from build123d import *

# Parameters (mm, degrees)
SKETCH2_R                      = 250
BOSS_EXTRUDE1_DEPTH            = 300
CUT_EXTRUDE1_DEPTH             = 464.680924775
CUT_EXTRUDE1_DEPTH_BACK        = 464.680924775
SKETCH3_W                      = 380
SKETCH3_H                      = 55
SHELL1_START                   = 140
SHELL1_OUTLINE_R               = 240
SHELL1_DEPTH                   = 150
SHELL1_START_2                 = 10
SHELL1_2_OUTLINE_R             = 240
SHELL1_2_DEPTH                 = 55
SHELL1_START_3                 = 65
SHELL1_3_DEPTH                 = 75
CUT_EXTRUDE2_REACH             = 546.885
SKETCH4_W                      = 120
SKETCH4_H                      = 20
CUT_EXTRUDE5_START             = -20
SKETCH6_R                      = 240
CUT_EXTRUDE5_DEPTH             = 20
CUT_EXTRUDE6_REACH             = 465.681
SKETCH8_3_W                    = 50
SKETCH8_3_H                    = 20
CUT_EXTRUDE6_DIRECTION_2_DEPTH = 464.680924775
CIRPATTERN1_COUNT              = 2
CIRPATTERN1_ANGLE              = 90
FILLET2_R                      = 30


# Read off the part's stored shape, not the designer's step: Shell1
with BuildPart() as part:
    # Sketch2 → Boss-Extrude1 (new body)
    with BuildSketch(Plane(origin=(0, 0, 0), x_dir=(1, 0, 0), z_dir=(0, 1, 0))):
        with Locations(Location((0, 0, 0), (0, 0, 270))):
            Circle(SKETCH2_R)
    extrude(amount=BOSS_EXTRUDE1_DEPTH)

    # Sketch3 → Cut-Extrude1 (cut, two sides: drawn at the far end of the back side and taken through both)
    with BuildSketch(Plane.XY.offset(-CUT_EXTRUDE1_DEPTH_BACK)):
        with Locations((-60, 102.5)):
            Rectangle(SKETCH3_W, SKETCH3_H)
    extrude(amount=CUT_EXTRUDE1_DEPTH + CUT_EXTRUDE1_DEPTH_BACK, mode=Mode.SUBTRACT)

    # Shell1 outline → Shell1 (cut)
    with BuildSketch(Plane(origin=(0, 0, 0), x_dir=(1, 0, 0), z_dir=(0, 1, 0)).offset(SHELL1_START)):
        Circle(SHELL1_OUTLINE_R)
    extrude(amount=SHELL1_DEPTH, mode=Mode.SUBTRACT)

    # Shell1 2 outline → Shell1 2 (cut)
    with BuildSketch(Plane(origin=(0, 0, 0), x_dir=(1, 0, 0), z_dir=(0, 1, 0)).offset(SHELL1_START_2)):
        Circle(SHELL1_2_OUTLINE_R)
    extrude(amount=SHELL1_2_DEPTH, mode=Mode.SUBTRACT)

    # Shell1 3 outline → Shell1 3 (cut)
    with BuildSketch(Plane(origin=(0, 0, 0), x_dir=(1, 0, 0), z_dir=(0, 1, 0)).offset(SHELL1_START_3)):
        with BuildLine():
            ThreePointArc((140, -194.935886896), (240, 0), (140, 194.935886896))
            Line((140, 194.935886896), (140, -194.935886896))
        make_face()
    extrude(amount=SHELL1_3_DEPTH, mode=Mode.SUBTRACT)

    # Sketch4 → Cut-Extrude2 (cut, up to next)
    with BuildSketch(Plane.ZY.offset(-130), mode=Mode.PRIVATE) as cut_extrude2_sk1:
        with Locations((0, 102.5)):
            Rectangle(SKETCH4_W, SKETCH4_H)
    cut_extrude2_tool1 = extrude(cut_extrude2_sk1.sketch, amount=-CUT_EXTRUDE2_REACH, mode=Mode.PRIVATE) & part.part
    add(cut_extrude2_tool1.solids().sort_by_distance((130, 102.5, 0))[0], mode=Mode.SUBTRACT)

    # Sketch6 → Cut-Extrude5 (cut)
    with BuildSketch(Plane(origin=(0, 300, 0), x_dir=(1, 0, 0), z_dir=(0, 1, 0)).offset(CUT_EXTRUDE5_START)):
        with Locations(Location((0, 0, 0), (0, 0, 270))):
            Circle(SKETCH6_R)
    extrude(amount=CUT_EXTRUDE5_DEPTH, mode=Mode.SUBTRACT)

    # Sketch8<3> → Cut-Extrude6 (cut, up to next)
    with BuildSketch(Plane(origin=(0, 0, 0), x_dir=(0, 0, -1), z_dir=(1, 0, 0)), mode=Mode.PRIVATE) as cut_extrude6_sk1:
        with Locations((0, 250)):
            Rectangle(SKETCH8_3_W, SKETCH8_3_H)
    cut_extrude6_tool1 = extrude(cut_extrude6_sk1.sketch, amount=-CUT_EXTRUDE6_REACH, mode=Mode.PRIVATE) & part.part
    cut_extrude6 = cut_extrude6_tool1.solids().sort_by_distance((0, 250, 0))[0]
    add(cut_extrude6, mode=Mode.SUBTRACT)

    # Sketch8<3> → Cut-Extrude6 direction 2 (cut)
    with BuildSketch(Plane(origin=(0, 0, 0), x_dir=(0, 0, -1), z_dir=(1, 0, 0))):
        with Locations((0, 250)):
            Rectangle(SKETCH8_3_W, SKETCH8_3_H)
    cut_extrude6_direction_2 = extrude(amount=CUT_EXTRUDE6_DIRECTION_2_DEPTH, mode=Mode.SUBTRACT)

    # CirPattern1: Cut-Extrude6, Cut-Extrude6 direction 2 ×2 about axis
    cirpattern1_axis = Axis((0, 300, 0), (0, 1, 0))
    add([cut_extrude6.rotate(cirpattern1_axis, i * CIRPATTERN1_ANGLE / (CIRPATTERN1_COUNT - 1)) for i in range(1, CIRPATTERN1_COUNT)], mode=Mode.SUBTRACT)
    add([cut_extrude6_direction_2.rotate(cirpattern1_axis, i * CIRPATTERN1_ANGLE / (CIRPATTERN1_COUNT - 1)) for i in range(1, CIRPATTERN1_COUNT)], mode=Mode.SUBTRACT)

    # Fillet2
    # the kernel refuses this fillet: 30 mm, written as the material it adds along each edge
    with BuildSketch(Plane(origin=(130, 130, -288.541565041), x_dir=(0, -1, 0), z_dir=(0, 0, 1))) as fillet2_piece_1_section:
        with BuildLine():
            CenterArc((FILLET2_R, -FILLET2_R), FILLET2_R, 90, 90)
            Line((0, -FILLET2_R), (0, 0))
            Line((0, 0), (FILLET2_R, 0))
        make_face()
    fillet2_piece_1 = extrude(amount=577.083130081, mode=Mode.PRIVATE)
    fillet2_piece_1 = fillet2_piece_1 & Plane(origin=(0, 108.141191738, 0), x_dir=(0, 0, 1), z_dir=(0, -1, 0)) * Cylinder(250, 1275, mode=Mode.PRIVATE)
    fillet2_piece_1 = split(fillet2_piece_1, bisect_by=Plane(origin=(129.633192853, 108.141191738, -60), z_dir=(0, 0, -1)), keep=Keep.TOP, mode=Mode.PRIVATE)
    fillet2_piece_1 = split(fillet2_piece_1, bisect_by=Plane(origin=(129.633192853, 112.5, -136.881350588), z_dir=(0, -1, 0)), keep=Keep.TOP, mode=Mode.PRIVATE)
    add(fillet2_piece_1)
    with BuildSketch(Plane(origin=(130, 130, -288.541565041), x_dir=(0, -1, 0), z_dir=(0, 0, 1))) as fillet2_piece_2_section:
        with BuildLine():
            CenterArc((FILLET2_R, -FILLET2_R), FILLET2_R, 90, 90)
            Line((0, -FILLET2_R), (0, 0))
            Line((0, 0), (FILLET2_R, 0))
        make_face()
    fillet2_piece_2 = extrude(amount=577.083130081, mode=Mode.PRIVATE)
    fillet2_piece_2 = fillet2_piece_2 & Plane(origin=(0, 124.602125162, 0), x_dir=(0, 0, 1), z_dir=(0, -1, 0)) * Cylinder(250, 1275, mode=Mode.PRIVATE)
    fillet2_piece_2 = split(fillet2_piece_2, bisect_by=Plane(origin=(122.496617269, 124.602125162, -60), z_dir=(0, 0, -1)), keep=Keep.TOP, mode=Mode.PRIVATE)
    fillet2_piece_2 = split(fillet2_piece_2, bisect_by=Plane(origin=(122.496617269, 112.5, -138.903095836), z_dir=(0, 1, 0)), keep=Keep.TOP, mode=Mode.PRIVATE)
    add(fillet2_piece_2)
    with BuildSketch(Plane(origin=(130, 130, -288.541565041), x_dir=(0, -1, 0), z_dir=(0, 0, 1))) as fillet2_piece_3_section:
        with BuildLine():
            CenterArc((FILLET2_R, -FILLET2_R), FILLET2_R, 90, 90)
            Line((0, -FILLET2_R), (0, 0))
            Line((0, 0), (FILLET2_R, 0))
        make_face()
    fillet2_piece_3 = extrude(amount=577.083130081, mode=Mode.PRIVATE)
    fillet2_piece_3 = split(fillet2_piece_3, bisect_by=Plane(origin=(122.639576661, 124.541490092, -60), z_dir=(0, 0, 1)), keep=Keep.TOP, mode=Mode.PRIVATE)
    fillet2_piece_3 = split(fillet2_piece_3, bisect_by=Plane(origin=(122.639576661, 124.541490092, 60), z_dir=(0, 0, -1)), keep=Keep.TOP, mode=Mode.PRIVATE)
    fillet2_piece_3 = split(fillet2_piece_3, bisect_by=Plane(origin=(122.639576661, 112.5, 0), z_dir=(0, 1, 0)), keep=Keep.TOP, mode=Mode.PRIVATE)
    add(fillet2_piece_3)
    with BuildSketch(Plane(origin=(130, 130, -288.541565041), x_dir=(0, -1, 0), z_dir=(0, 0, 1))) as fillet2_piece_4_section:
        with BuildLine():
            CenterArc((FILLET2_R, -FILLET2_R), FILLET2_R, 90, 90)
            Line((0, -FILLET2_R), (0, 0))
            Line((0, 0), (FILLET2_R, 0))
        make_face()
    fillet2_piece_4 = extrude(amount=577.083130081, mode=Mode.PRIVATE)
    fillet2_piece_4 = fillet2_piece_4 & Plane(origin=(0, 108.141191737, 0), x_dir=(0, 0, 1), z_dir=(0, -1, 0)) * Cylinder(250, 1275, mode=Mode.PRIVATE)
    fillet2_piece_4 = split(fillet2_piece_4, bisect_by=Plane(origin=(129.633192853, 108.141191737, 60), z_dir=(0, 0, 1)), keep=Keep.TOP, mode=Mode.PRIVATE)
    fillet2_piece_4 = split(fillet2_piece_4, bisect_by=Plane(origin=(129.633192853, 112.5, 136.881350585), z_dir=(0, -1, 0)), keep=Keep.TOP, mode=Mode.PRIVATE)
    add(fillet2_piece_4)
    with BuildSketch(Plane(origin=(130, 130, -288.541565041), x_dir=(0, -1, 0), z_dir=(0, 0, 1))) as fillet2_piece_5_section:
        with BuildLine():
            CenterArc((FILLET2_R, -FILLET2_R), FILLET2_R, 90, 90)
            Line((0, -FILLET2_R), (0, 0))
            Line((0, 0), (FILLET2_R, 0))
        make_face()
    fillet2_piece_5 = extrude(amount=577.083130081, mode=Mode.PRIVATE)
    fillet2_piece_5 = fillet2_piece_5 & Plane(origin=(0, 124.602106632, 0), x_dir=(0, 0, 1), z_dir=(0, -1, 0)) * Cylinder(250, 1275, mode=Mode.PRIVATE)
    fillet2_piece_5 = split(fillet2_piece_5, bisect_by=Plane(origin=(122.496572682, 124.602106632, 60), z_dir=(0, 0, 1)), keep=Keep.TOP, mode=Mode.PRIVATE)
    fillet2_piece_5 = split(fillet2_piece_5, bisect_by=Plane(origin=(122.496572682, 112.5, 138.903516263), z_dir=(0, 1, 0)), keep=Keep.TOP, mode=Mode.PRIVATE)
    add(fillet2_piece_5)
    with BuildSketch(Plane(origin=(130, 75, -288.541565041), x_dir=(-1, 0, 0), z_dir=(0, 0, 1))) as fillet2_piece_6_section:
        with BuildLine():
            CenterArc((FILLET2_R, -FILLET2_R), FILLET2_R, 90, 90)
            Line((0, -FILLET2_R), (0, 0))
            Line((0, 0), (FILLET2_R, 0))
        make_face()
    fillet2_piece_6 = extrude(amount=577.083130081, mode=Mode.PRIVATE)
    fillet2_piece_6 = fillet2_piece_6 & Plane(origin=(0, 80.397884307, 0), x_dir=(0, 0, 1), z_dir=(0, -1, 0)) * Cylinder(250, 1275, mode=Mode.PRIVATE)
    fillet2_piece_6 = split(fillet2_piece_6, bisect_by=Plane(origin=(122.496621968, 80.397884307, -60), z_dir=(0, 0, -1)), keep=Keep.TOP, mode=Mode.PRIVATE)
    fillet2_piece_6 = split(fillet2_piece_6, bisect_by=Plane(origin=(122.496621968, 92.5, -138.903256412), z_dir=(0, -1, 0)), keep=Keep.TOP, mode=Mode.PRIVATE)
    add(fillet2_piece_6)
    with BuildSketch(Plane(origin=(130, 75, -288.541565041), x_dir=(-1, 0, 0), z_dir=(0, 0, 1))) as fillet2_piece_7_section:
        with BuildLine():
            CenterArc((FILLET2_R, -FILLET2_R), FILLET2_R, 90, 90)
            Line((0, -FILLET2_R), (0, 0))
            Line((0, 0), (FILLET2_R, 0))
        make_face()
    fillet2_piece_7 = extrude(amount=577.083130081, mode=Mode.PRIVATE)
    fillet2_piece_7 = fillet2_piece_7 & Plane(origin=(0, 96.858808254, 0), x_dir=(0, 0, 1), z_dir=(0, -1, 0)) * Cylinder(250, 1275, mode=Mode.PRIVATE)
    fillet2_piece_7 = split(fillet2_piece_7, bisect_by=Plane(origin=(129.633192853, 96.858808254, -60), z_dir=(0, 0, -1)), keep=Keep.TOP, mode=Mode.PRIVATE)
    fillet2_piece_7 = split(fillet2_piece_7, bisect_by=Plane(origin=(129.633192853, 92.5, -136.881350463), z_dir=(0, 1, 0)), keep=Keep.TOP, mode=Mode.PRIVATE)
    add(fillet2_piece_7)
    with BuildSketch(Plane(origin=(130, 75, -288.541565041), x_dir=(-1, 0, 0), z_dir=(0, 0, 1))) as fillet2_piece_8_section:
        with BuildLine():
            CenterArc((FILLET2_R, -FILLET2_R), FILLET2_R, 90, 90)
            Line((0, -FILLET2_R), (0, 0))
            Line((0, 0), (FILLET2_R, 0))
        make_face()
    fillet2_piece_8 = extrude(amount=577.083130081, mode=Mode.PRIVATE)
    fillet2_piece_8 = split(fillet2_piece_8, bisect_by=Plane(origin=(122.639576661, 80.458509908, -60), z_dir=(0, 0, 1)), keep=Keep.TOP, mode=Mode.PRIVATE)
    fillet2_piece_8 = split(fillet2_piece_8, bisect_by=Plane(origin=(122.639576661, 92.5, 0), z_dir=(0, -1, 0)), keep=Keep.TOP, mode=Mode.PRIVATE)
    fillet2_piece_8 = split(fillet2_piece_8, bisect_by=Plane(origin=(122.639576661, 80.458509908, 60), z_dir=(0, 0, -1)), keep=Keep.TOP, mode=Mode.PRIVATE)
    add(fillet2_piece_8)
    with BuildSketch(Plane(origin=(130, 75, -288.541565041), x_dir=(-1, 0, 0), z_dir=(0, 0, 1))) as fillet2_piece_9_section:
        with BuildLine():
            CenterArc((FILLET2_R, -FILLET2_R), FILLET2_R, 90, 90)
            Line((0, -FILLET2_R), (0, 0))
            Line((0, 0), (FILLET2_R, 0))
        make_face()
    fillet2_piece_9 = extrude(amount=577.083130081, mode=Mode.PRIVATE)
    fillet2_piece_9 = fillet2_piece_9 & Plane(origin=(0, 80.397869734, 0), x_dir=(0, 0, 1), z_dir=(0, -1, 0)) * Cylinder(250, 1275, mode=Mode.PRIVATE)
    fillet2_piece_9 = split(fillet2_piece_9, bisect_by=Plane(origin=(122.496641232, 92.5, 138.903074765), z_dir=(0, -1, 0)), keep=Keep.TOP, mode=Mode.PRIVATE)
    fillet2_piece_9 = split(fillet2_piece_9, bisect_by=Plane(origin=(122.496641232, 80.397869734, 60), z_dir=(0, 0, 1)), keep=Keep.TOP, mode=Mode.PRIVATE)
    add(fillet2_piece_9)
    with BuildSketch(Plane(origin=(130, 75, -288.541565041), x_dir=(-1, 0, 0), z_dir=(0, 0, 1))) as fillet2_piece_10_section:
        with BuildLine():
            CenterArc((FILLET2_R, -FILLET2_R), FILLET2_R, 90, 90)
            Line((0, -FILLET2_R), (0, 0))
            Line((0, 0), (FILLET2_R, 0))
        make_face()
    fillet2_piece_10 = extrude(amount=577.083130081, mode=Mode.PRIVATE)
    fillet2_piece_10 = fillet2_piece_10 & Plane(origin=(0, 96.858808255, 0), x_dir=(0, 0, 1), z_dir=(0, -1, 0)) * Cylinder(250, 1275, mode=Mode.PRIVATE)
    fillet2_piece_10 = split(fillet2_piece_10, bisect_by=Plane(origin=(129.633192854, 92.5, 136.881350462), z_dir=(0, 1, 0)), keep=Keep.TOP, mode=Mode.PRIVATE)
    fillet2_piece_10 = split(fillet2_piece_10, bisect_by=Plane(origin=(129.633192854, 96.858808255, 60), z_dir=(0, 0, 1)), keep=Keep.TOP, mode=Mode.PRIVATE)
    add(fillet2_piece_10)


solid = part.part
Work out the finished part from the listing and answer in its coordinate system (mm). A direction names the side the tool comes from. Give positions to 0.01 mm unless a question says otherwise; leave off trailing zeros. Loops run counter-clockwise (first coordinate to the right, second up) from the corner with the lowest first, then second, coordinate; pieces in that order, holes last. Notation, with made-up numbers: (38.25, 89.5) -> (65.25, 89.5) arc R25 ccw to (65.25, 122.5) -> close; hole circle Ø2 at (-25, 86). An arc over 180 degrees is marked (long way). Use a Markdown table: item, result. Add a question column.
1. Find the intervals of material crossed by probe 1 along Y at (x, z) = (22.5, 78.5); probe 2 along X at (y, z) = (138.5, 0); probe 3 along Y at (x, z) = (-174, -171.5), in increasing order.
2. For faces 1 (the flat face through (134, 112.5, -1)), 2 (the cylindrical face through (120.08, 82.71, -3.21)), 3 (the cylindrical face through (211.61, 120.75, 113.23)), 4 (the flat face through (4, 0, -3)), 5 (the flat face through (223, 300, -94)), determine the directions among +Z, -Z, +X, -X, +Y, -Y from which every point of the face is accessible in a straight line to the end or side of a thin tool.
3. Flat-ended cylindrical pins translate along their axes: pin 1 Ø1 at (x, y) = (86, 269.5) entering from -Z (3 decimals); pin 2 Ø3 at (x, y) = (134, 154.5) entering from -Z; pin 3 Ø12 at (y, z) = (43, 196.5) entering from +X; pin 4 Ø1 at (x, z) = (127, -180) entering from -Y. Find the tip coordinate at first contact, or state that the pin passes through.
4. Section B-B on z = 0 is taken. Determine the outline of the cut face in (x, y).
5. Section A-A on x = 0 is taken. Determine the outline of the cut face in (y, z).
6. Section C-C on x = -126.5 is taken. Determine the outline of the cut face in (y, z), and give its area (3 significant figures).
7. Section D-D on y = 269.5 is taken. Determine the outline of the cut face in (x, z), and give its area (3 significant figures).
8. Determine the mould class of faces 6 (the flat face through (-3, 10, -3)), 7 (the flat face through (134, 92.5, 1)), 8 (the flat face through (140, 119, -3)), 9 (the flat face through (-53, 140, -3)) for opening direction Y: released by +Y, released by -Y, zero draft, split by the parting line, or undercut.
Results below:
| question | item | result |
|---|---|---|
| 1 | probe 1 | y = 0 to 10, 65 to 75, 130 to 140 |
| 1 | probe 2 | x = -250 to 140, 240 to 250 |
| 1 | probe 3 | y = 0 to 75, 130 to 300 |
| 2 | face 1 | -X |
| 2 | face 2 | +Z, -Z, -X |
| 2 | face 3 | none |
| 2 | face 4 | +Z, -Z, +X, -X, -Y |
| 2 | face 5 | +Z, -Z, +X, -X, +Y |
| 3 | pin 1 | stops at z = -234.925 |
| 3 | pin 2 | stops at z = -212 |
| 3 | pin 3 | stops at x = 161.89 |
| 3 | pin 4 | stops at y = 0 |
| 4 | outline | (-250, 0) -> (250, 0) -> (250, 240) -> (240, 240) -> (240, 10) -> (-240, 10) -> (-240, 65) -> (140, 65) -> (140, 92.5) -> (127.27, 92.5) arc R30 cw to (100, 75) -> (-250, 75) -> close; (-250, 130) -> (100, 130) arc R30 cw to (127.27, 112.5) -> (140, 112.5) -> (140, 140) -> (-240, 140) -> (-240, 240) -> (-250, 240) -> close; (-250, 260) -> (-240, 260) -> (-240, 300) -> (-250, 300) -> close; (240, 260) -> (250, 260) -> (250, 300) -> (240, 300) -> close |
| 5 | outline | (0, -250) -> (75, -250) -> (75, 250) -> (0, 250) -> close; (130, -250) -> (240, -250) -> (240, -240) -> (140, -240) -> (140, 240) -> (240, 240) -> (240, 250) -> (130, 250) -> close; (260, -250) -> (300, -250) -> (300, -240) -> (260, -240) -> close; (260, 240) -> (300, 240) -> (300, 250) -> (260, 250) -> close; hole (10, -240) -> (65, -240) -> (65, 240) -> (10, 240) -> close |
| 6 | outline | (0, -215.63) -> (75, -215.63) -> (75, 215.63) -> (0, 215.63) -> close; (130, -215.63) -> (300, -215.63) -> (300, -203.96) -> (140, -203.96) -> (140, 203.96) -> (300, 203.96) -> (300, 215.63) -> (130, 215.63) -> close; hole (10, -203.96) -> (65, -203.96) -> (65, 203.96) -> (10, 203.96) -> close |
| 6 | area | 18,000 mm^2 |
| 7 | outline | circle Ø500 at (0, 0); hole circle Ø480 at (0, 0) |
| 7 | area | 15,400 mm^2 |
| 8 | face 6 | undercut |
| 8 | face 7 | undercut |
| 8 | face 8 | zero draft |
| 8 | face 9 | released by +Y |
